from build123d import *

# Parameters (mm, degrees)
F1_DEPTH = 50
F2_R     = 2
F3_DEPTH = 10
F4_R     = 1


with BuildPart() as f1:
    # F0 (on Front) → F1 (new body, symmetric)
    with BuildSketch(Plane.XZ):
        with BuildLine():
            ThreePointArc((4.5, 0), (1.5, -4.242641), (-3.5, -2.828427))
            Line((-3.5, -2.828427), (-3.5, -7))
            Line((-3.5, -7), (10.5, -7))
            Line((10.5, -7), (10.5, 3))
            Line((10.5, 3), (4.5, 3))
            Line((4.5, 3), (4.5, 0))
        make_face()
    extrude(amount=F1_DEPTH, both=True)

    # F2 (on face) → F3 (cut, through all)
    with BuildSketch(Plane.XY.offset(3)):
        with Locations((6.6, -40)):
            Circle(F2_R)
        with Locations((6.6, 40)):
            Circle(F2_R)
    extrude(amount=-F3_DEPTH, mode=Mode.SUBTRACT)

    # F4
    f4_edges = [f1.edges().sort_by_distance(p)[0] for p in [
        (10.5, 0, -7),
        (10.5, 50, -2),
        (10.5, 0, 3),
        (10.5, -50, -2),
        (1.5, -50, -4.242641),
        (-3.5, -50, -4.914214),
        (3.5, -50, -7),
        (7.5, -50, 3),
        (4.5, -50, 1.5),
        (-3.5, 0, -2.828427),
        (-3.5, 0, -7),
    ]]
    fillet(f4_edges, radius=F4_R)


solid = f1.part
Here's how the part is built. I have some questions about the finished solid (model axes, mm). A direction names the side the tool comes from. Coordinates: 2 decimals unless noted, no trailing zeros. Write each loop counter-clockwise with the first axis right and the second up, starting at its lowest first coordinate (ties: lowest second). Pieces come first, ordered by that corner, then holes. Notation, with made-up numbers: (57, 28.5) - (99, 28.5) arc R30 cw to (99, 50.5) - close; hole circle Ø3 at (52, 50). An arc over 180 degrees is marked (long way). Use one line per item in the form item = value.
1) I need wall thicknesses on line 1 (Y direction, x = 6.6, z = -3.25); line 2 (Y direction, x = 5.5, z = 1.25); line 3 (X direction, y = -19, z = 1). Which ranges of each line are inside material? Lowest first, please.
Solved:
line_1 = -50 to -42, -38 to 38, 42 to 50
line_2 = -50 to -41.67, -38.33 to 38.33, 41.67 to 50
line_3 = 4.5 to 10.5
2) On a 3-axis mill with a long thin cutter (end or side, diameter ignored), from which of +Z, -Z, +X, -X, +Y, -Y can I reach the whole of each face in a straight line? I mean faces 4 (the flat face through (10.5, -1, -2)), 5 (the flat face through (4.5, 0, 2)). Say none if no direction works.
Solved:
face_4 = +Z, -Z, +X, +Y, -Y
face_5 = +Z, -X, +Y, -Y
3) Suppose I cut it at D-D, the plane z = -1.25. Give the number of separate pieces and of enclosed holes in the cut face, plus the area to 3 significant figures.
Solved:
separate_pieces = 1
enclosed_holes = 2
area = 592 mm2
4) Thinking about a two-plate mould opening in Y: for faces 1 (the cylindrical face through (2.405, -0.193, -3.804)), 2 (the flat face through (4, 50, -3)), 3 (the cylindrical face through (7.523, 38.226, -1.93)), which applies, released by +Y, released by -Y, zero draft, split by the parting line, or undercut?
Solved:
face_1 = zero draft
face_2 = released by +Y
face_3 = undercut
5) I'm going to push flat-ended pins straight in: P1, Ø2, axis at x = 2.5, y = 7.5, coming from the +Z side; P2, Ø6.5, axis at x = 6.6, y = -40, coming from the -Z side; P3, Ø0.9, axis at y = 2, z = 2, coming from the -X side; P4, Ø3, axis at x = -0.5, y = 20.5, coming from the +Z side. Where does each tip first touch, or does it pass through?
Solved:
P1 = -2.83
P2 = -7
P3 = 4.5
P4 = -4.03
6) Suppose I cut it at A-A, the plane x = 6.6. Write out the boundary of the cut face in (y, z).
Solved:
outline = (-50, -6) arc R1 ccw to (-49, -7) - (-42, -7) - (-42, 3) - (-49, 3) arc R1 ccw to (-50, 2) - close; (-38, -7) - (38, -7) - (38, 3) - (-38, 3) - close; (42, -7) - (50, -7) - (50, 3) - (42, 3) - close
7) Suppose I cut it at C-C, the plane y = 27.5. Write out the boundary of the cut face in (x, z), plus the area to 3 significant figures.
Solved:
outline = (-3.5, -6) arc R1 ccw to (-2.5, -7) - (9.5, -7) arc R1 ccw to (10.5, -6) - (10.5, 2) arc R1 ccw to (9.5, 3) - (4.5, 3) - (4.5, 0) arc R4.5 cw to (-2.05, -4.01) arc R1 ccw to (-3.5, -4.9) - close
area = 84.7 mm2
8) Suppose I cut it at B-B, the plane y = 40. Write out the boundary of the cut face in (x, z), plus the area to 3 significant figures.
Solved:
outline = (-3.5, -6) arc R1 ccw to (-2.5, -7) - (4.6, -7) - (4.6, 3) - (4.5, 3) - (4.5, 0) arc R4.5 cw to (-2.05, -4.01) arc R1 ccw to (-3.5, -4.9) - close; (8.6, -7) - (9.5, -7) arc R1 ccw to (10.5, -6) - (10.5, 2) arc R1 ccw to (9.5, 3) - (8.6, 3) - close
area = 44.7 mm2
